Part model, mm, in its own coordinate system. A direction names the side the tool comes from. Give positions to 0.01 mm unless a question says otherwise; leave off trailing zeros. Write each loop counter-clockwise with the first axis right and the second up, starting at its lowest first coordinate (ties: lowest second). Pieces come first, ordered by that corner, then holes.
```python
from build123d import *

# Parameters (mm, degrees)
F0_W     = 40
F0_H     = 35
F1_DEPTH = 10
F2_W     = 40
F2_H     = 30
F3_DEPTH = 5
F4_W     = 1
F4_H     = 2
F5_DEPTH = 40
F6_R     = 1
F7_DEPTH = 4
F9_DEPTH = 4


with BuildPart() as f1:
    # F0 (on Front) → F1 (new body)
    with BuildSketch(Plane.XZ):
        Rectangle(F0_W, F0_H)
    extrude(amount=F1_DEPTH)

    # F2 (on face) → F3 (cut)
    with BuildSketch(Plane.XZ.offset(10)):
        with Locations((0, 2.5)):
            Rectangle(F2_W, F2_H)
    extrude(amount=-F3_DEPTH, mode=Mode.SUBTRACT)

    # F4 (on face) → F5 (join, through all)
    with BuildSketch(Plane.YZ.offset(20)):
        with Locations((-9.5, -11.5)):
            Rectangle(F4_W, F4_H)
    extrude(amount=-F5_DEPTH)

    # F6 (on face) → F7 (join)
    with BuildSketch(Plane.XZ.offset(5)):
        with Locations((-1.07176, 4.339809)):
            Circle(F6_R)
        with Locations((-5.244032, 1.778612)):
            Circle(F6_R)
    extrude(amount=F7_DEPTH)

    # F8 (on face) → F9 (join)
    with BuildSketch(Plane.XZ.offset(5)):
        Polygon((-20, -12.5), (20, -12.5), (20, -8.5), (19, -8.5), (17, -8.5), (15, -8.5), (13, -8.5), (11, -8.5), (9, -8.5), (7, -8.5), (5, -8.5), (3, -8.5), (1, -8.5), (-1, -8.5), (-3, -8.5), (-5, -8.5), (-7, -8.5), (-9, -8.5), (-11, -8.5), (-13, -8.5), (-15, -8.5), (-17, -8.5), (-19, -8.5), (-20, -8.5), align=None)
        Polygon((17, -8.5), (19, -8.5), (18.7, -6.5), (18, -6.5), (17.3, -6.5), align=None)
        Polygon((-18.7, -6.5), (-19, -8.5), (-17, -8.5), (-17.3, -6.5), (-18, -6.5), align=None)
        Polygon((13, -8.5), (15, -8.5), (14.7, -6.5), (14, -6.5), (13.3, -6.5), align=None)
        Polygon((-14.7, -6.5), (-15, -8.5), (-13, -8.5), (-13.3, -6.5), (-14, -6.5), align=None)
        Polygon((9, -8.5), (11, -8.5), (10.7, -6.5), (10, -6.5), (9.3, -6.5), align=None)
        Polygon((-10.7, -6.5), (-11, -8.5), (-9, -8.5), (-9.3, -6.5), (-10, -6.5), align=None)
        Polygon((5, -8.5), (7, -8.5), (6.7, -6.5), (6, -6.5), (5.3, -6.5), align=None)
        Polygon((-6.7, -6.5), (-7, -8.5), (-5, -8.5), (-5.3, -6.5), (-6, -6.5), align=None)
        Polygon((1, -8.5), (3, -8.5), (2.7, -6.5), (2, -6.5), (1.3, -6.5), align=None)
        Polygon((-2.7, -6.5), (-3, -8.5), (-1, -8.5), (-1.3, -6.5), (-2, -6.5), align=None)
    extrude(amount=F9_DEPTH)


with BuildPart() as f10_1:
    # F10: copy of F1
    add(f1.part)


solid = f10_1.part
```
1) Saw through at A-A, the plane x = 15.5. Write the cut outline in (y, z).
Answers follow:
outline: (-10, -17.5) - (0, -17.5) - (0, 17.5) - (-5, 17.5) - (-5, -8.5) - (-9, -8.5) - (-9, -10.5) - (-10, -10.5) - close
2) Saw through at D-D, the plane z = 12.5. Write the cut outline in (x, y), then the cut area to 3 significant figures.
Answers follow:
outline: (-20, -5) - (20, -5) - (20, 0) - (-20, 0) - close
area: 200 mm2
3) Saw through at B-B, the plane x = -10. Write the cut outline in (y, z), then the cut area to 3 significant figures.
Answers follow:
outline: (-10, -17.5) - (0, -17.5) - (0, 17.5) - (-5, 17.5) - (-5, -6.5) - (-9, -6.5) - (-9, -10.5) - (-10, -10.5) - close
area: 226 mm2
4) Saw through at C-C, the plane y = -6.5. Count the separate pieces of the cut face and the enclosed holes in it, then the cut area to 3 significant figures.
Answers follow:
separate pieces: 3
enclosed holes: 0
area: 400 mm2
5) Pin check, flat tips, straight feed: pin 1 Ø1.1 at (x, y) = (-18, -6.5) entering from +Z; pin 2 Ø1.6 at (x, y) = (4, -7) entering from +Z; pin 3 Ø1 at (x, z) = (-1.5, 4.5) entering from -Y. Stop position of each tip, or through.
Answers follow:
pin 1: stops at z = -6.5
pin 2: stops at z = -8.5
pin 3: stops at y = -9
6) Wall check: L1, parallel to Y at x = 9, z = -10; L2, parallel to Y at x = -17, z = -2; L3, parallel to Z at x = 2.5, y = -7. Give the ranges that are in metal, low to high.
Answers follow:
L1: y = -9 to 0
L2: y = -5 to 0
L3: z = -17.5 to -6.5
7) Two-plate mould, pull along Z, no slides. Class faces 1 (the face through (20, -4, -4)), 2 (the face through (14, -7, -6.5)), 3 (the face through (0, -7, -8.5)): +Z half, -Z half, draft (parallel to the pull), parting line (faces both ways), or undercut.
Answers follow:
face 1: draft
face 2: +Z half
face 3: undercut
8) 3-axis set-ups, long thin cutter, end or side, ignore diameter. For faces 4 (the face through (-10, -7, -6.5)), 5 (the face through (-2, -7, -6.5)), 6 (the face through (1.15, -6.97, -7.49)), 7 (the face through (-5.15, -6.97, -7.51)): which of +Z, -Z, +X, -X, +Y, -Y reach the whole face in a straight line?
Answers follow:
face 4: +Z, +X, -X, -Y
face 5: +X, -X, -Y
face 6: +Z, -Y
face 7: -Y
